Input: dimensioned drawing with shaded views. Units: mm. Origin: part minimum x, y, z. A direction names the side the tool comes from. Give positions to 0.01 mm unless a question says otherwise; leave off trailing zeros. Order: outer loops, then holes, each group sorted by start corner. A loop starts at its lowest first (then second) coordinate and runs counter-clockwise, first axis right, second up.
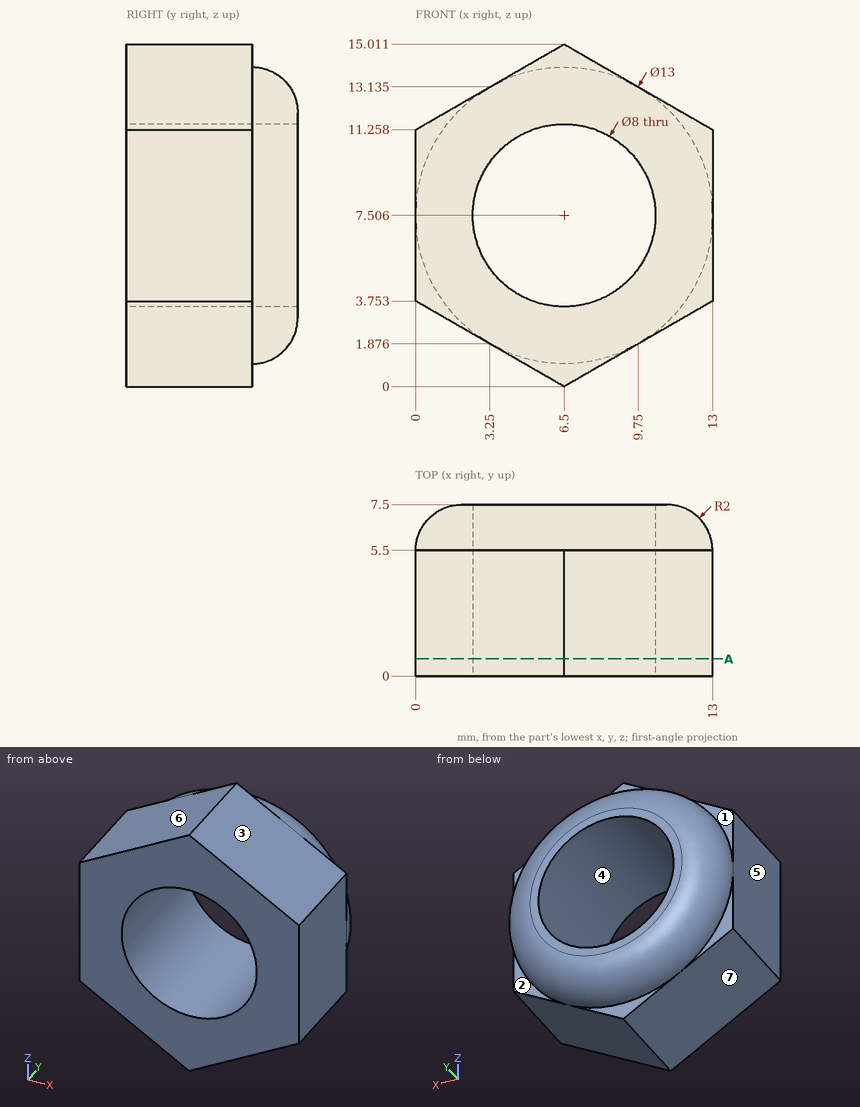
1) Reachability of the marked faces 1, 2 and 3 from +Z, -Z, +X, -X, +Y, -Y: full face, straight path, thin tool, end or side. Return the list, or none.
Report:
face 1: +Z, -X, +Y
face 2: -Z, +X, +Y
face 3: +Z, +X, +Y, -Y
2) Draft query along Z for the marked faces 4, 5, 6 and 7. Return one class per face: +Z half, -Z half, draft (parallel to the pull), parting line (faces both ways), or undercut.
Report:
face 4: undercut
face 5: draft
face 6: +Z half
face 7: -Z half
3) Material intervals for L1, parallel to X at y = 6, z = 4.75 (1 decimal); L2, parallel to X at y = 6.25, z = 7 (1 decimal); L3, parallel to Z at x = 9.5, y = 1.25, sorted ascending.
Report:
L1: x = 0.7 to 3.6, 9.4 to 12.3
L2: x = 0.2 to 2.5, 10.5 to 12.8
L3: z = 1.73 to 4.86, 10.15 to 13.28
4) Section query A-A, the plane y = 0.75. Return the cut outline in (x, z) (1 decimal).
Report:
outline: (0, 3.8) - (6.5, 0) - (13, 3.8) - (13, 11.3) - (6.5, 15) - (0, 11.3) - close; hole circle Ø8 at (6.5, 7.5)
5) Pin query (flat end, axial travel): pin 1 (2.5 mm diameter, centred on x = 11.5, z = 9.5, fed in from +Y); pin 2 (0.6 mm diameter, centred on x = 6, z = 0.5, fed in from +Y); pin 3 (1.5 mm diameter, centred on x = 7.5, z = 14, fed in from +Y). Return the tip coordinate at first contact, or that it passes through.
Report:
pin 1: stops at y = 7.5
pin 2: stops at y = 5.5
pin 3: stops at y = 7
